from build123d import *

# Parameters (mm, degrees)
F0_W     = 177.8
F0_H     = 152.4
F1_DEPTH = 12.7
F2_W     = 50.8
F2_H     = 50.8
F2_W_2   = 38.1
F2_H_2   = 38.1
F3_DEPTH = 609.6


with BuildPart() as f1:
    # F0 (on Top) → F1 (new body)
    with BuildSketch(Plane.XY):
        with Locations((88.9, 76.2)):
            Rectangle(F0_W, F0_H)
    extrude(amount=F1_DEPTH)

    # F2 (on face) → F3 (join)
    with BuildSketch(Plane(origin=(0, 0, 0), x_dir=(1, 0, 0), z_dir=(0, 0, -1))):
        with Locations((88.9, -76.2)):
            Rectangle(F2_W, F2_H)
        with Locations((88.9, -76.2)):
            Rectangle(F2_W_2, F2_H_2, mode=Mode.SUBTRACT)
    extrude(amount=F3_DEPTH)


solid = f1.part
The listing builds one solid part. Answer for the finished solid, in the listing's coordinates (mm). A direction names the side the tool comes from. Coordinates: 2 decimals unless noted, no trailing zeros. Loops run counter-clockwise (first coordinate to the right, second up) from the corner with the lowest first, then second, coordinate; pieces in that order, holes last. Notation, with made-up numbers: (-29.5, 89.25) -> (28.5, 89.25) arc R21 cw to (28.5, 98.25) -> close; hole circle Ø5 at (22, 47). An arc over 180 degrees is marked (long way). Write item = value, one per line. Start each with the question number.
1) Straight lines are drawn through the part: line 1 (X direction, y = 90.5, z = -278); line 2 (Z direction, x = 44, y = 109); line 3 (Y direction, x = 91, z = -522.5). For each, find the intervals that lie inside material, in ascending order. Write a range as from..to.
2) The mould has two halves that part along X. Classify faces 5 (the face through (107.95, 76, -301)), 6 (the face through (89, 95.25, -301)), 7 (the face through (89, 101.6, -301)), 8 (the face through (177.8, 75, 6)): released by +X, released by -X, zero draft, split by the parting line, or undercut.
3) A cutting plane is placed at B-B (y = 73.5). Give the vertices of the cut face in (x, z), then the cut area to 4 significant figures.
4) A cutting plane is placed at D-D (y = 32.5). Give the vertices of the cut face in (x, z), then the cut area to 3 significant figures.
5) A cutting plane is placed at A-A (z = -242). Give the vertices of the cut face in (x, y).
6) A tool of negligible diameter and unlimited length cuts with its end or side. For faces 1 (the face through (114.3, 77, -301)), 2 (the face through (63.5, 77, -301)), 3 (the face through (89, 76, 0)), 4 (the face through (89, 50.8, -301)), from which of +Z, -Z, +X, -X, +Y, -Y can it reach the whole face along a straight path? Write none if from no direction.
7) Given pin 1 Ø3 at (x, y) = (24, 105) entering from -Z; pin 2 Ø8 at (y, z) = (51, -544) entering from -X; pin 3 Ø6 at (y, z) = (89, -283.5) entering from +X, each flat-ended and moving along its own axis, determine where each tip first touches the part or whether it passes through.
8) A cutting plane is placed at C-C (x = 85). Give the vertices of the cut face in (y, z), then the cut area to 3 significant figures.
Responses:
q1.line_1 = 63.5..69.85, 107.95..114.3
q1.line_2 = 0..12.7
q1.line_3 = 50.8..57.15, 95.25..101.6
q2.face_5 = undercut
q2.face_6 = undercut
q2.face_7 = zero draft
q2.face_8 = released by +X
q3.outline = (0, 0) -> (63.5, 0) -> (63.5, -609.6) -> (69.85, -609.6) -> (69.85, 0) -> (107.95, 0) -> (107.95, -609.6) -> (114.3, -609.6) -> (114.3, 0) -> (177.8, 0) -> (177.8, 12.7) -> (0, 12.7) -> close
q3.area = 10,000 mm²
q4.outline = (0, 0) -> (177.8, 0) -> (177.8, 12.7) -> (0, 12.7) -> close
q4.area = 2,260 mm²
q5.outline = (63.5, 50.8) -> (114.3, 50.8) -> (114.3, 101.6) -> (63.5, 101.6) -> close; hole (69.85, 57.15) -> (107.95, 57.15) -> (107.95, 95.25) -> (69.85, 95.25) -> close
q6.face_1 = -Z, +X, +Y, -Y
q6.face_2 = -Z, -X, +Y, -Y
q6.face_3 = -Z
q6.face_4 = -Z, +X, -X, -Y
q7.pin_1 = 0
q7.pin_2 = 63.5
q7.pin_3 = 114.3
q8.outline = (0, 0) -> (50.8, 0) -> (50.8, -609.6) -> (57.15, -609.6) -> (57.15, 0) -> (95.25, 0) -> (95.25, -609.6) -> (101.6, -609.6) -> (101.6, 0) -> (152.4, 0) -> (152.4, 12.7) -> (0, 12.7) -> close
q8.area = 9,680 mm²
